from build123d import *

# Parameters (mm, degrees)
IZIM1_R                     = 25
Y_KSEKLIK_EKSTR_ZYON1_DEPTH = 35
IZIM2_R                     = 6.5
KES_EKSTR_ZYON1_DEPTH       = 30
IZIM3_R                     = 2.5
KES_EKSTR_ZYON2_DEPTH       = 3
IZIM4_R                     = 1.5
KES_EKSTR_ZYON3_DEPTH       = 49.363209157


with BuildPart() as part:
    # Çizim1 → Yükseklik-Ekstrüzyon1 (new body)
    with BuildSketch(Plane(origin=(0, 0, 0), x_dir=(1, 0, 0), z_dir=(0, 1, 0))):
        with Locations(Location((0, 0, 0), (0, 0, 270))):
            Circle(IZIM1_R)
    extrude(amount=Y_KSEKLIK_EKSTR_ZYON1_DEPTH)

    # Çizim2 → Kes-Ekstrüzyon1 (cut)
    with BuildSketch(Plane(origin=(0, 35, 0), x_dir=(1, 0, 0), z_dir=(0, 1, 0))):
        with Locations(Location((0, 0, 0), (0, 0, 270))):
            Circle(IZIM2_R)
    extrude(amount=-KES_EKSTR_ZYON1_DEPTH, mode=Mode.SUBTRACT)

    # Çizim3 → Kes-Ekstrüzyon2 (cut)
    with BuildSketch(Plane(origin=(0, 5, 0), x_dir=(1, 0, 0), z_dir=(0, 1, 0))):
        with Locations(Location((0, 0, 0), (0, 0, 270))):
            Circle(IZIM3_R)
    extrude(amount=-KES_EKSTR_ZYON2_DEPTH, mode=Mode.SUBTRACT)

    # Çizim4 → Kes-Ekstrüzyon3 (cut, through all)
    with BuildSketch(Plane(origin=(0, 2, 0), x_dir=(1, 0, 0), z_dir=(0, 1, 0))):
        with Locations(Location((0, 0, 0), (0, 0, 270))):
            Circle(IZIM4_R)
    extrude(amount=-KES_EKSTR_ZYON3_DEPTH, mode=Mode.SUBTRACT)


solid = part.part
Verification items for the finished model (mm, model axes). A direction names the side the tool comes from. Give positions to 0.01 mm unless a question says otherwise; leave off trailing zeros. Loops run counter-clockwise (first coordinate to the right, second up) from the corner with the lowest first, then second, coordinate; pieces in that order, holes last.
1) Depth check by flat-ended pin: pin 1 Ø1 at (y, z) = (13, -0.5) entering from -X; pin 2 Ø10.5 at (x, z) = (0, 0) entering from -Y; pin 3 Ø6 at (y, z) = (28.5, 18.5) entering from -X; pin 4 Ø5 at (y, z) = (27.5, 7) entering from -X. Enter the tip coordinate at first touch or a pass-through.
2) Set-up check for faces 4 (the flat face through (-5, 35, 5)), 5 (the cylindrical face through (-3.955, 20.21, -5.158)): record each of +Z, -Z, +X, -X, +Y, -Y from which the full face is reachable in a straight line by a thin tool's end or side.
3) Draft check along Z on faces 1 (the cylindrical face through (7.509, 17.255, 23.846)), 2 (the flat face through (-2, 2, 0)), 3 (the flat face through (-5, 0, 0)). Enter one of: pulls with the +Z half, pulls with the -Z half, needs draft (parallel to the pull), parting line crosses it, or undercut.
4) Thickness scan on line 1 along X through (y, z) = (3.2, 0); line 2 along X through (y, z) = (21.25, 0); line 3 along Z through (x, y) = (3, 25). Record the ranges inside material, lowest first.
5) Sectioned sample at D-D, the plane z = -15. Enter the section's corners in (x, y), then the cut area to 3 significant figures.
6) Sectioned sample at C-C, the plane y = 24. Enter the section's corners in (x, z).
7) Sectioned sample at B-B, the plane x = 0. Enter the section's corners in (y, z), then the cut area to 3 significant figures.
8) Sectioned sample at A-A, the plane z = 0. Enter the section's corners in (x, y), then the cut area to 3 significant figures.
Answers:
1. pin 1: stops at x = -25
1. pin 2: stops at y = 0
1. pin 3: stops at x = -19.62
1. pin 4: stops at x = -24.59
2. face 4: +Z, -Z, +X, -X, +Y
2. face 5: +Y
3. face 1: parting line crosses it
3. face 2: undercut
3. face 3: needs draft
4. line 1: x = -25 to -2.5, 2.5 to 25
4. line 2: x = -25 to -6.5, 6.5 to 25
4. line 3: z = -24.82 to -5.77, 5.77 to 24.82
5. outline: (-20, 0) - (20, 0) - (20, 35) - (-20, 35) - close
5. area: 1,400 mm2
6. outline: circle Ø50 at (0, 0); hole circle Ø13 at (0, 0)
7. outline: (0, -25) - (35, -25) - (35, -6.5) - (5, -6.5) - (5, -2.5) - (2, -2.5) - (2, -1.5) - (0, -1.5) - close; (0, 1.5) - (2, 1.5) - (2, 2.5) - (5, 2.5) - (5, 6.5) - (35, 6.5) - (35, 25) - (0, 25) - close
7. area: 1,340 mm2
8. outline: (-25, 0) - (-1.5, 0) - (-1.5, 2) - (-2.5, 2) - (-2.5, 5) - (-6.5, 5) - (-6.5, 35) - (-25, 35) - close; (1.5, 0) - (25, 0) - (25, 35) - (6.5, 35) - (6.5, 5) - (2.5, 5) - (2.5, 2) - (1.5, 2) - close
8. area: 1,340 mm2
